Geometry: final body of the model. Coordinates: model frame, mm. Give positions to 0.01 mm unless a question says otherwise; leave off trailing zeros. Write each loop counter-clockwise with the first axis right and the second up, starting at its lowest first coordinate (ties: lowest second). Pieces come first, ordered by that corner, then holes. Notation, with made-up numbers: (46, 73) - (78, 73) arc R33 cw to (78, 110) - close; hole circle Ø4 at (-23, 2.5). An arc over 180 degrees is marked (long way). Return JSON: item names as keys, results as strings.
from build123d import *

# Parameters (mm, degrees)
SKETCH1_W           = 400
SKETCH1_H           = 500
BOSS_EXTRUDE1_DEPTH = 4
CUT_EXTRUDE1_REACH  = 6
SKETCH3_W           = 292
SKETCH3_H           = 392
SKETCH6_R           = 2.5
CUT_EXTRUDE3_DEPTH  = 4
SKETCH7_R           = 3
CUT_EXTRUDE4_DEPTH  = 4


with BuildPart() as part:
    # Sketch1 → Boss-Extrude1 (new body)
    with BuildSketch(Plane.XY):
        with Locations((200, 250)):
            Rectangle(SKETCH1_W, SKETCH1_H)
    extrude(amount=BOSS_EXTRUDE1_DEPTH)

    # Sketch3 → Cut-Extrude1 (cut, up to next)
    with BuildSketch(Plane.XY.offset(4), mode=Mode.PRIVATE) as cut_extrude1_sk1:
        with Locations((200, 250)):
            Rectangle(SKETCH3_W, SKETCH3_H)
    cut_extrude1_tool1 = extrude(cut_extrude1_sk1.sketch, amount=-CUT_EXTRUDE1_REACH, mode=Mode.PRIVATE) & part.part
    add(cut_extrude1_tool1.solids().sort_by_distance((200, 250, 4))[0], mode=Mode.SUBTRACT)

    # Sketch6 → Cut-Extrude3 (cut)
    with BuildSketch(Plane.XY.offset(4)):
        with Locations((355.5, 83.5)):
            Circle(SKETCH6_R)
        with Locations((355.5, 115.5)):
            Circle(SKETCH6_R)
        with Locations((355.5, 175.5)):
            Circle(SKETCH6_R)
        with Locations((355.5, 207.5)):
            Circle(SKETCH6_R)
    cut_extrude3 = extrude(amount=-CUT_EXTRUDE3_DEPTH, mode=Mode.SUBTRACT)

    # Mirror1: Cut-Extrude3 across plane
    add(cut_extrude3.mirror(Plane(origin=(200, 0, 0), x_dir=(0, 0, 1), z_dir=(1, 0, 0))), mode=Mode.SUBTRACT)

    # Sketch7 → Cut-Extrude4 (cut)
    with BuildSketch(Plane.XY.offset(4)):
        with Locations((375, 475)):
            Circle(SKETCH7_R)
        with Locations((25, 475)):
            Circle(SKETCH7_R)
        with Locations((25, 25)):
            Circle(SKETCH7_R)
        with Locations((375, 25)):
            Circle(SKETCH7_R)
    extrude(amount=-CUT_EXTRUDE4_DEPTH, mode=Mode.SUBTRACT)


solid = part.part
Q1. Material intervals for probe 1 along Y at (x, z) = (44.5, 3); probe 2 along X at (y, z) = (207.5, 1); probe 3 along X at (y, z) = (190, 0.4), sorted ascending. Write a range as [from, to].
Answer key:
{"probe 1": "y = [0, 81], [86, 113], [118, 173], [178, 205], [210, 500]", "probe 2": "x = [0, 42], [47, 54], [346, 353], [358, 400]", "probe 3": "x = [0, 54], [346, 400]"}
Q2. Section query A-A, the plane y = 342.5. Return the cut outline in (x, z).
Answer key:
{"outline": "(0, 0) - (54, 0) - (54, 4) - (0, 4) - close; (346, 0) - (400, 0) - (400, 4) - (346, 4) - close"}
Q3. Section query B-B, the plane z = 1.85. Count the separate pieces of the cut face and the enclosed holes in it, plus the area to 3 significant figures.
Answer key:
{"separate pieces": "1", "enclosed holes": "13", "area": "85,300 mm^2"}
Q4. Pin query (flat end, axial travel): P1, Ø6.5, axis at x = 355.5, y = 115.5, coming from the -Z side. Return the tip coordinate at first contact, or that it passes through.
Answer key:
{"P1": "stops at z = 0"}
Q5. Section query C-C, the plane x = 230. Return the cut outline in (y, z), plus the area to 3 significant figures.
Answer key:
{"outline": "(0, 0) - (54, 0) - (54, 4) - (0, 4) - close; (446, 0) - (500, 0) - (500, 4) - (446, 4) - close", "area": "432 mm^2"}
